Autodesk Inventor part; units mm, degrees
ref_plane "YZ Plane" through (0, 0, 0) normal (1, 0, 0) x (0, 1, 0)
ref_plane "XZ Plane" through (0, 0, 0) normal (0, 1, 0) x (-1, 0, 0)
ref_plane "XY Plane" through (0, 0, 0) normal (0, 0, 1) x (1, 0, 0)
sketch "スケッチ1" plane through (0, 0, 0) normal (0, 1, 0) x (-1, 0, 0)
  line L0 (0, 0) -> (60, 0)
  line L1 (60, 0) -> (60, -60)
  line L2 (60, -60) -> (0, -60)
  line L3 (0, -60) -> (0, 0)
  dimension "d0" = 60
  dimension "d1" = 60
extrude "押し出し1" add sketch "スケッチ1" along normal blind 80
chamfer "面取り1" distance 5 distance2 50 1 edges at (0, 80, -30) measured on face at (-20, 80, -40)
chamfer "面取り2" distance 5 distance2 50 1 edges at (-60, 80, -30) measured on face at (-23.3333, 80, -40)
chamfer "面取り3" distance 5 distance2 50 1 edges at (-30, 80, -60) measured on face at (-21.6667, 80, -40)
chamfer "面取り4" distance 5 distance2 50 1 edges at (-30, 80, 0) measured on face at (-21.6667, 80, -18.3333)
fillet "フィレット1" radius 5 12 edges at (0, 15, -60) (-60, 15, -60) (-60, 15, 0) (0, 15, 0) (-57.5, 55, -2.5) (-57.5, 55, -57.5) (-55, 80, -30) (-30, 80, -5) (-5, 80, -30) (-30, 80, -55) (-2.5, 55, -2.5) (-2.5, 55, -57.5)
sketch "スケッチ2" plane through (0, 0, 0) normal (0, -1, 0) x (1, 0, 0)
  line L0 (-60, -55) -> (-60, -5)
  line L1 (-60, -30) -> (0, -30) construction
  line L2 (0, -5) -> (0, -55)
  line L3 (-55, -19.95) -> (-5, -19.95)
  line L4 (-5, -19.95) -> (-5, -40.05)
  line L5 (-5, -40.05) -> (-55, -40.05)
  line L6 (-55, -40.05) -> (-55, -19.95)
  line L7 (-55, -19.95) -> (-5, -40.05) construction
  line L8 (-5, -19.95) -> (-55, -40.05) construction
  point P0 (0, 0)
  point P1 (-30, -30)
  dimension "d17" = 50
  dimension "d18" = 20.1
extrude "押し出し2" cut sketch "スケッチ2" against normal blind 1
properties part number "raida-"
CAD build for the part. Positions are in the model's coordinates, mm. Give positions to 0.01 mm unless a question says otherwise; leave off trailing zeros. Write each loop counter-clockwise with the first axis right and the second up, starting at its lowest first coordinate (ties: lowest second). Pieces come first, ordered by that corner, then holes. Notation, with made-up numbers: M 75,83.5 L 111,83.5 A19 ccw 111,89.5 Z; hole C -12.75,6 d10. An arc over 180 degrees is marked long. Put each result on its own line as item: value. Start each with the question number.
(1) Probe L1, parallel to Y at x = -30, z = -26.5; L2, parallel to Y at x = -52, z = -7.5; L3, parallel to Z at x = -39.5, y = 47.5. List the from-to ranges inside material, lowest first.
(2) Band-saw the part on A-A, the plane x = -19. Write the cut outline in (y, z), and give its area (3 significant figures).
(3) Band-saw the part on B-B, the plane z = -45. Write the cut outline in (x, y).
(4) Flat gauge pins, fed straight in: pin 1 Ø3 at (x, y) = (-45, 39.5) entering from +Z; pin 2 Ø6 at (x, z) = (-39.5, -34.5) entering from -Y; pin 3 Ø1.5 at (y, z) = (56.5, -33) entering from +X (3 decimals). Where does each tip first touch, or does it go through?
(5) Band-saw the part on C-C, the plane z = -26.5. Write the cut outline in (x, y), and give its area (3 significant figures).
(6) Mould opens along Z. For faces 1 (the face through (-2, 15, -59)), 2 (the face through (-30, 0, -16)), 3 (the face through (-30, 1, -30)) say: +Z half, -Z half, draft (parallel to the pull), parting line (faces both ways), or undercut.
Response values:
1. L1: y = 1 to 80
1. L2: y = 0 to 79.31
1. L3: z = -58.25 to -1.75
2. outline: M 0,-60 L 30,-60 L 75.5,-55.45 A5 ccw 80,-50.48 L 80,-9.52 A5 ccw 75.5,-4.55 L 30,0 L 0,0 L 0,-19.95 L 1,-19.95 L 1,-40.05 L 0,-40.05 Z
2. area: 4,520 mm2
3. outline: M -60,0 L 0,0 L 0,30 L -4.55,75.5 A5 ccw -9.52,80 L -50.48,80 A5 ccw -55.45,75.5 L -60,30 Z
4. pin 1: stops at z = -0.8
4. pin 2: stops at y = 1
4. pin 3: stops at x = -2.575
5. outline: M -60,0 L -55,0 L -55,1 L -5,1 L -5,0 L 0,0 L 0,30 L -4.55,75.5 A5 ccw -9.52,80 L -50.48,80 A5 ccw -55.45,75.5 L -60,30 Z
5. area: 4,490 mm2
6. face 1: -Z half
6. face 2: draft
6. face 3: undercut
